Check sheet for the drawn part. Datum: minimum x, y, z corner. Units: mm. A direction names the side the tool comes from. Give positions to 0.01 mm unless a question says otherwise; leave off trailing zeros. Loops run counter-clockwise (first coordinate to the right, second up) from the corner with the lowest first, then second, coordinate; pieces in that order, holes last.
1. Go/stop test with flat-tipped pins: pin 1 Ø10 at (x, z) = (129, 116.5) entering from +Y (3 decimals); pin 2 Ø1 at (x, y) = (133.5, 65) entering from +Z; pin 3 Ø2 at (y, z) = (75, 110) entering from -X; pin 4 Ø15.5 at (y, z) = (95.5, 51) entering from +X. Record where each tip stops, or that it passes through.
2. Material ranges on L1, parallel to Y at x = 61, z = 137.5 (3 decimals); L2, parallel to X at y = 58.5, z = 60; L3, parallel to X at y = 60, z = 44.5, recorded low to high.
3. Release check for a two-part mould opening along Y. For the marked faces 4, 5 and 6 record: +Y half, -Y half, draft (parallel to the pull), parting line (faces both ways), or undercut.
4. Tool access check on the marked faces 1, 2 and 3. Record the directions out of +Z, -Z, +X, -X, +Y, -Y that give a thin tool (end or side, any length) a straight path to the whole face; none if there is none.
5. Cross-section at C-C, the plane z = 92. Record the cut outline in (x, y) (3 decimals).
6. Cross-section at B-B, the plane x = 101. Record the cut outline in (y, z) (3 decimals), plus the area to 3 significant figures.
7. Cross-section at A-A, the plane y = 79. Record the cut outline in (x, z).
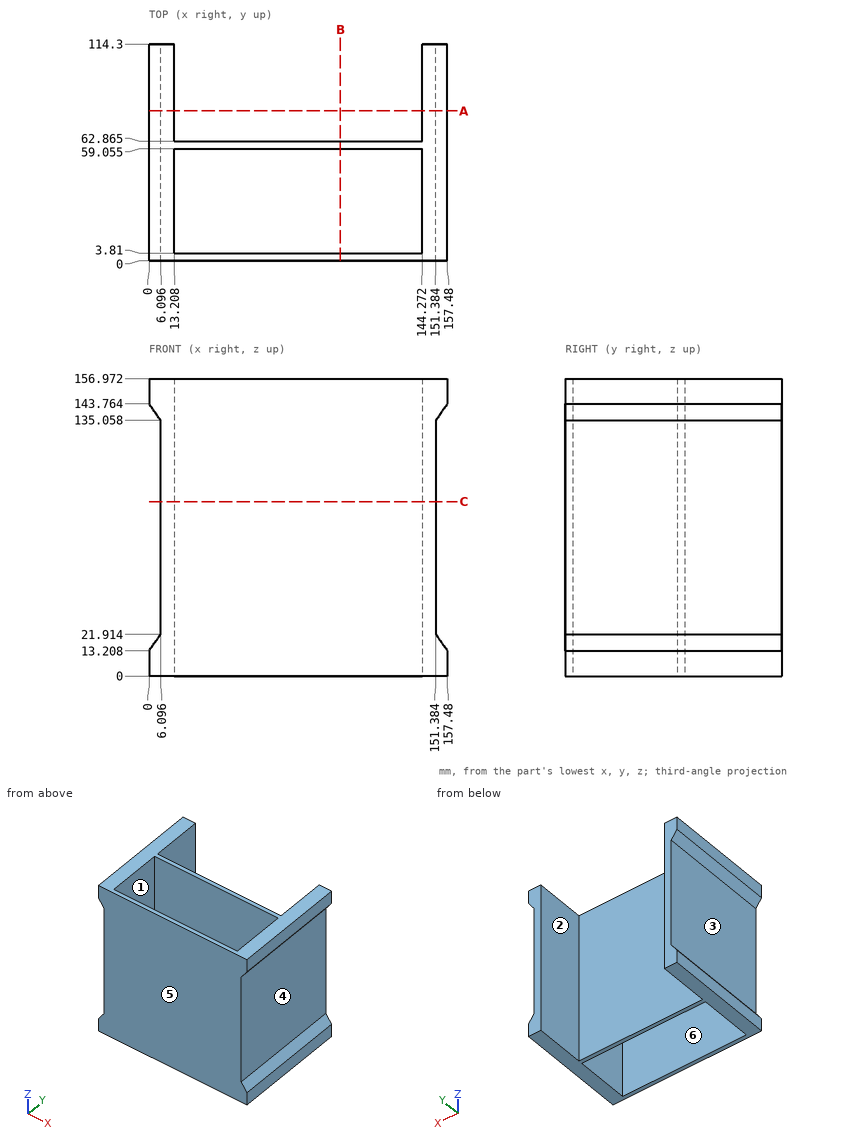
Result:
1. pin 1: stops at y = 62.865
1. pin 2: passes through
1. pin 3: stops at x = 6.1
1. pin 4: stops at x = 151.38
2. L1: y = 0 to 3.81, 59.055 to 62.865
2. L2: x = 6.1 to 13.21, 144.27 to 151.38
2. L3: x = 6.1 to 151.38
3. face 4: draft
3. face 5: -Y half
3. face 6: undercut
4. face 1: +Z, -Z
4. face 2: +Z, -Z, +Y
4. face 3: -X, +Y, -Y
5. outline: (6.096, 0) - (151.384, 0) - (151.384, 114.3) - (144.272, 114.3) - (144.272, 62.865) - (13.208, 62.865) - (13.208, 114.3) - (6.096, 114.3) - close; hole (13.208, 3.81) - (144.272, 3.81) - (144.272, 59.055) - (13.208, 59.055) - close
6. outline: (0, 0) - (3.81, 0) - (3.81, 156.972) - (0, 156.972) - close; (59.055, 0) - (62.865, 0) - (62.865, 156.972) - (59.055, 156.972) - close
6. area: 1,200 mm2
7. outline: (0, 0) - (13.21, 0) - (13.21, 156.97) - (0, 156.97) - (0, 143.76) - (6.1, 135.06) - (6.1, 21.91) - (0, 13.21) - close; (144.27, 0) - (157.48, 0) - (157.48, 13.21) - (151.38, 21.91) - (151.38, 135.06) - (157.48, 143.76) - (157.48, 156.97) - (144.27, 156.97) - close
